from build123d import *

# Parameters (mm, degrees)
BOSS_EXTRU_1_DEPTH      = 50
TROU_TARAUD_M61_D       = 5
ESQUISSE4_W             = 2
ESQUISSE4_H             = 50
BOSS_EXTRU_2_DEPTH      = 1
ESQUISSE5_R             = 10
ENL_V_MAT_EXTRU_1_DEPTH = 64.716654463


with BuildPart() as part:
    # Esquisse1 → Boss.-Extru.1 (new body)
    with BuildSketch(Plane.XY):
        with BuildLine():
            Line((-36.108337762, 0), (-36.108337762, 15))
            Line((-36.108337762, 15), (13.891662238, 15))
            Line((13.891662238, 15), (13.891662238, 0))
            Line((13.891662238, 0), (5, 0))
            ThreePointArc((5, 0), (0, 5), (-5, 0))
            Line((-5, 0), (-36.108337762, 0))
        make_face()
    extrude(amount=BOSS_EXTRU_1_DEPTH)

    # Trou taraudé M61 (through all)
    with Locations(Plane(origin=(0, 0, 0), x_dir=(-1, 0, 0), z_dir=(0, -1, 0))):
        with Locations((12.056043545, -42.065822787), (28.108337762, -8)):
            Hole(TROU_TARAUD_M61_D / 2)

    # Esquisse4 → Boss.-Extru.2 (add)
    with BuildSketch(Plane.XZ):
        with Locations((-35.108337762, 25)):
            Rectangle(ESQUISSE4_W, ESQUISSE4_H)
    extrude(amount=BOSS_EXTRU_2_DEPTH)

    # Esquisse5 → Enlèv. mat.-Extru.1 (cut, through all)
    with BuildSketch(Plane(origin=(0, 15, 0), x_dir=(1, 0, 0), z_dir=(0, 1, 0))):
        with Locations(Location((-21.108337762, -25, 0), (0, 0, 270))):
            Circle(ESQUISSE5_R)
    extrude(amount=-ENL_V_MAT_EXTRU_1_DEPTH, mode=Mode.SUBTRACT)


solid = part.part
Check sheet for the modelled part. Datum: model origin and axes. Units: mm. A direction names the side the tool comes from. Give positions to 0.01 mm unless a question says otherwise; leave off trailing zeros. Loops run counter-clockwise (first coordinate to the right, second up) from the corner with the lowest first, then second, coordinate; pieces in that order, holes last. Notation, with made-up numbers: M -18,-24 L -9,-24 A11 ccw -9,-15 Z; hole C -39.75,89 d4. An arc over 180 degrees is marked long. Return JSON: item names as keys, results as strings. Group by question number.
1. Go/stop test with flat-tipped pins: pin 1 (1.5 mm diameter, centred on x = -14.5, z = 32, fed in from -Y); pin 2 (0.5 mm diameter, centred on y = -0.5, z = 30, fed in from +X). Record where each tip stops, or that it passes through.
2. Mould release check, pull along X, two halves, no side actions. Record for faces 1 (the cylindrical face through (-18.105, 7.605, 34.538)), 2 (the flat face through (-36.108, 7, 25)), 3 (the flat face through (-11, 7, 0)): released by +X, released by -X, zero draft, split by the parting line, or undercut.
3. Cross-section at D-D on z = 38. Record the boundary of the cut face in (x, y).
4. Cross-section at C-C on y = 4.25. Record the boundary of the cut face in (x, z).
5. Tool access check on faces 4 (the flat face through (10, 0, 25)), 5 (the flat face through (-11, 7, 50)). Record the directions out of +Z, -Z, +X, -X, +Y, -Y that give a thin tool (end or side, any length) a straight path to the whole face; none if there is none.
6. Cross-section at A-A on z = 25. Record the boundary of the cut face in (x, y).
7. Cross-section at B-B on x = -17.5. Record the boundary of the cut face in (y, z).
8. Thickness scan on L1, parallel to X at y = 5.5, z = 8; L2, parallel to X at y = 8.5, z = 25; L3, parallel to Z at x = -28, y = 9.5. Record the ranges inside material, lowest first.
Return value:
{
 "1": {"pin 1": "y = 0", "pin 2": "x = -34.11"},
 "2": {"face 1": "undercut", "face 2": "released by -X", "face 3": "zero draft"},
 "3": {"outline": "M -36.11,-1 L -34.11,-1 L -34.11,0 L -5,0 A5 cw 5,0 L 13.89,0 L 13.89,15 L -36.11,15 Z"},
 "4": {"outline": "M -36.11,0 L -2.63,0 L -2.63,50 L -36.11,50 Z; M 2.63,0 L 13.89,0 L 13.89,50 L 2.63,50 Z; hole C -21.11,25 d20; hole C -28.11,8 d5; hole C -12.06,42.07 d5"},
 "5": {"face 4": "+Z, -Z, +X, -Y", "face 5": "+Z, +X, -X, +Y, -Y"},
 "6": {"outline": "M -36.11,-1 L -34.11,-1 L -34.11,0 L -31.11,0 L -31.11,15 L -36.11,15 Z; M -11.11,0 L -5,0 A5 cw 5,0 L 13.89,0 L 13.89,15 L -11.11,15 Z"},
 "7": {"outline": "M 0,0 L 15,0 L 15,15.67 L 0,15.67 Z; M 0,34.33 L 15,34.33 L 15,50 L 0,50 Z"},
 "8": {"L1": "-36.11 to -30.61, -25.61 to 13.89", "L2": "-36.11 to -31.11, -11.11 to 13.89", "L3": "0 to 5.5, 10.5 to 17.75, 32.25 to 50"}
}
